from build123d import *

# Parameters (mm, degrees)
SKETCH1_W            = 40
SKETCH1_H            = 30
SKETCH1_R            = 6.25
BODY_DEPTH           = 2
SKETCH2_W            = 40
SKETCH2_H            = 30
SKETCH2_R            = 8.3
BEARINGS_PLACE_DEPTH = 3
SKETCH3_R            = 1.85
INSERTS_PLACE_DEPTH  = 4


with BuildPart() as part:
    # Sketch1 → Body (new body)
    with BuildSketch(Plane(origin=(0, 0, 0), x_dir=(1, 0, 0), z_dir=(0, 1, 0))):
        Rectangle(SKETCH1_W, SKETCH1_H)
        with Locations(Location((0, 0, 0), (0, 0, 270))):
            Circle(SKETCH1_R, mode=Mode.SUBTRACT)
    extrude(amount=BODY_DEPTH)

    # Sketch2 → Bearings_Place (add)
    with BuildSketch(Plane(origin=(0, 2, 0), x_dir=(1, 0, 0), z_dir=(0, 1, 0))):
        Rectangle(SKETCH2_W, SKETCH2_H)
        with Locations(Location((0, 0, 0), (0, 0, 270))):
            Circle(SKETCH2_R, mode=Mode.SUBTRACT)
    extrude(amount=BEARINGS_PLACE_DEPTH)

    # Sketch3 → Inserts_Place (cut)
    with BuildSketch(Plane(origin=(0, 5, 0), x_dir=(1, 0, 0), z_dir=(0, 1, 0))):
        with Locations(Location((-10, 10, 0), (0, 0, 270))):
            Circle(SKETCH3_R)
        with Locations(Location((10, 10, 0), (0, 0, 270))):
            Circle(SKETCH3_R)
        with Locations(Location((10, -10, 0), (0, 0, 270))):
            Circle(SKETCH3_R)
        with Locations(Location((-10, -10, 0), (0, 0, 270))):
            Circle(SKETCH3_R)
    extrude(amount=-INSERTS_PLACE_DEPTH, mode=Mode.SUBTRACT)


solid = part.part
Design review of the part built by this model. Coordinates are the model's own, in mm. A direction names the side the tool comes from. Coordinates: 2 decimals unless noted, no trailing zeros. Order: outer loops, then holes, each group sorted by start corner. A loop starts at its lowest first (then second) coordinate and runs counter-clockwise, first axis right, second up. Notation, with made-up numbers: (22, 32) - (66, 32) arc R20 cw to (66, 42) - close; hole circle Ø9 at (31.5, 46). An arc over 180 degrees is marked (long way). Put each result on its own line as item: value.
1) Take a section at A-A, the plane z = 0. Give the boundary of the cut face in (x, y), and give its area (3 significant figures).
Response values:
outline: (-20, 0) - (-6.25, 0) - (-6.25, 2) - (-8.3, 2) - (-8.3, 5) - (-20, 5) - close; (6.25, 0) - (20, 0) - (20, 5) - (8.3, 5) - (8.3, 2) - (6.25, 2) - close
area: 125 mm²
2) Take a section at D-D, the plane x = 10. Give the boundary of the cut face in (y, z), and give its area (3 significant figures).
Response values:
outline: (0, -15) - (5, -15) - (5, -11.85) - (1, -11.85) - (1, -8.15) - (5, -8.15) - (5, 8.15) - (1, 8.15) - (1, 11.85) - (5, 11.85) - (5, 15) - (0, 15) - close
area: 120 mm²
3) Take a section at C-C, the plane z = -10. Give the boundary of the cut face in (x, y), and give its area (3 significant figures).
Response values:
outline: (-20, 0) - (20, 0) - (20, 5) - (11.85, 5) - (11.85, 1) - (8.15, 1) - (8.15, 5) - (-8.15, 5) - (-8.15, 1) - (-11.85, 1) - (-11.85, 5) - (-20, 5) - close
area: 170 mm²
4) The part is to be moulded in two halves that separate along Z. For faces 3 (the face through (-3, 2, -6)), 4 (the face through (0, 2, 15)), 5 (the face through (0, 2, -15)), 6 (the face through (20, 2, 0)), say which applies: released by +Z, released by -Z, zero draft, split by the parting line, or undercut.
Response values:
face 3: undercut
face 4: released by +Z
face 5: released by -Z
face 6: zero draft
5) Wall thickness on L1, parallel to X at y = 2.3, z = 10; L2, parallel to X at y = 3.15, z = 7.5; L3, parallel to Y at x = -2, z = -6.5: over which ranges is each line inside the solid? List them lowest first. Write a range as from..to.
Response values:
L1: x = -20..-11.85, -8.15..8.15, 11.85..20
L2: x = -20..-3.56, 3.56..20
L3: y = 0..2
6) Tool access review of faces 1 (the face through (9.29, 3.03, 11.71)), 2 (the face through (0, 0, -7)): name each direction out of +Z, -Z, +X, -X, +Y, -Y from which nothing blocks a thin tool from reaching the whole face with its end or side.
Response values:
face 1: +Y
face 2: +Z, -Z, +X, -X, -Y
7) Insertion check: P1, Ø1.5, axis at x = -6.5, z = 6, coming from the -Y side; P2, Ø2, axis at x = 10, z = 10, coming from the +Y side. Each pin has a flat end and moves straight along its axis. Give the tip position at first contact, or say it passes through.
Response values:
P1: stops at y = 0
P2: stops at y = 1
8) Take a section at B-B, the plane x = 0. Give the boundary of the cut face in (y, z), and give its area (3 significant figures).
Response values:
outline: (0, -15) - (5, -15) - (5, -8.3) - (2, -8.3) - (2, -6.25) - (0, -6.25) - close; (0, 6.25) - (2, 6.25) - (2, 8.3) - (5, 8.3) - (5, 15) - (0, 15) - close
area: 75.2 mm²
